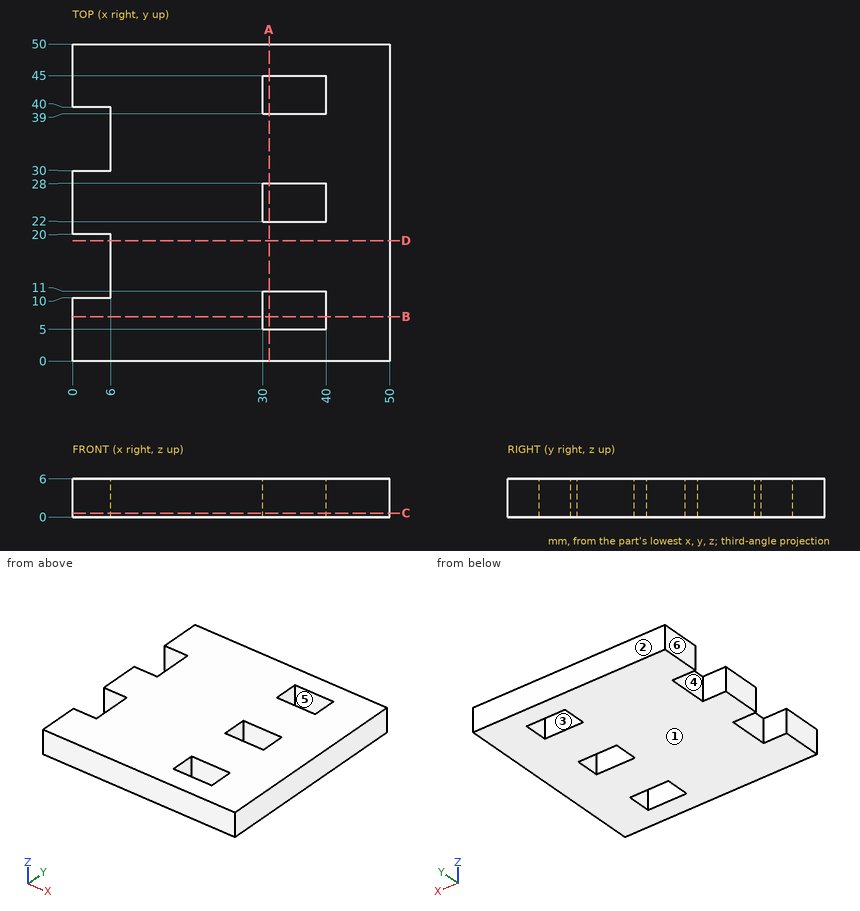
Part print with two shaded views. Sizes in mm from the minimum x, y, z corner. A direction names the side the tool comes from. Coordinates: 2 decimals unless noted, no trailing zeros. Write each loop counter-clockwise with the first axis right and the second up, starting at its lowest first coordinate (ties: lowest second). Pieces come first, ordered by that corner, then holes.
(1) Cut at D-D on y = 19. List the corners of the cut face in (x, z), and give its area (3 significant figures).
(2) Cut at C-C on z = 0.6. List the corners of the cut face in (x, y), and give its area (3 significant figures).
(3) Cut at B-B on y = 7. List the corners of the cut face in (x, z), and give its area (3 significant figures).
(4) 3-axis set-ups, long thin cutter, end or side, ignore diameter. For the marked faces 4, 5 and 6: which of +Z, -Z, +X, -X, +Y, -Y reach the whole face in a straight line?
(5) Drill centre lines: line 1 (Y direction, x = 5, z = 2.95); line 2 (Y direction, x = 34.5, z = 0.8); line 3 (X direction, y = 43, z = 4.45). Where is each one in solid material? Low to high.
(6) Cut at A-A on x = 31. List the corners of the cut face in (y, z).
(7) Pin check, flat tip, straight feed: pin 1 Ø1.8 at (y, z) = (13.5, 4) entering from -X. Stop position of the tip, or through.
(8) Mould opens along Y. For the marked faces 1, 2 and 3 say: pulls with the +Y half, pulls with the -Y half, needs draft (parallel to the pull), parting line crosses it, or undercut.
Working result:
1. outline: (6, 0) - (50, 0) - (50, 6) - (6, 6) - close
1. area: 264 mm2
2. outline: (0, 0) - (50, 0) - (50, 50) - (0, 50) - (0, 40) - (6, 40) - (6, 30) - (0, 30) - (0, 20) - (6, 20) - (6, 10) - (0, 10) - close; hole (30, 5) - (40, 5) - (40, 11) - (30, 11) - close; hole (30, 22) - (40, 22) - (40, 28) - (30, 28) - close; hole (30, 39) - (40, 39) - (40, 45) - (30, 45) - close
2. area: 2,200 mm2
3. outline: (0, 0) - (30, 0) - (30, 6) - (0, 6) - close; (40, 0) - (50, 0) - (50, 6) - (40, 6) - close
3. area: 240 mm2
4. face 4: +Z, -Z, -X
4. face 5: +Z, -Z
4. face 6: +Z, -Z, -X, +Y, -Y
5. line 1: y = 0 to 10, 20 to 30, 40 to 50
5. line 2: y = 0 to 5, 11 to 22, 28 to 39, 45 to 50
5. line 3: x = 0 to 30, 40 to 50
6. outline: (0, 0) - (5, 0) - (5, 6) - (0, 6) - close; (11, 0) - (22, 0) - (22, 6) - (11, 6) - close; (28, 0) - (39, 0) - (39, 6) - (28, 6) - close; (45, 0) - (50, 0) - (50, 6) - (45, 6) - close
7. pin 1: stops at x = 6
8. face 1: needs draft
8. face 2: pulls with the +Y half
8. face 3: undercut
